CAD build for the part. Positions are in the model's coordinates, mm. Face numbers are marked on the shaded views. A direction names the side the tool comes from. Give positions to 0.01 mm unless a question says otherwise; leave off trailing zeros. Loops run counter-clockwise (first coordinate to the right, second up) from the corner with the lowest first, then second, coordinate; pieces in that order, holes last. Notation, with made-up numbers: (-27.5, 18.25) -> (7.5, 18.25) arc R35 ccw to (7.5, 52.25) -> close; hole circle Ø8 at (-24, -26). An arc over 180 degrees is marked (long way). Write each question's results on one line, items separated by ' | '. Start each with the question number.
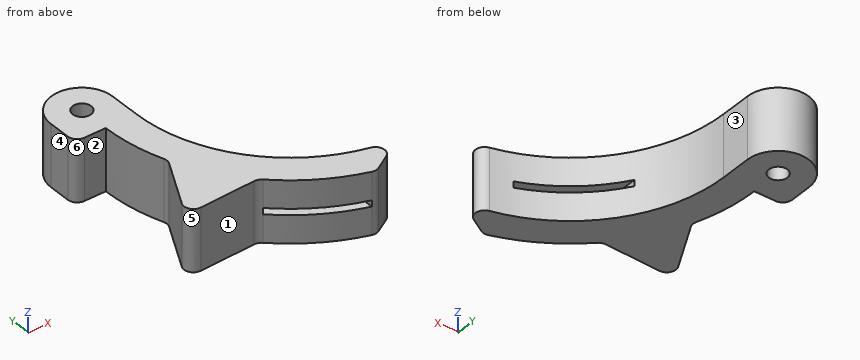
```python
from build123d import *

# Parameters (mm, degrees)
SKETCH_2_R              = 1.5
EXTRUDE_1_DEPTH         = 10
FILLET_1_R              = 1.5
CUT_EXTRUDE_START       = 8.978636738
CUT_EXTRUDE_6_OUTLINE_W = 18
CUT_EXTRUDE_6_OUTLINE_H = 1
CUT_EXTRUDE_6_DEPTH     = 12.065744551


# Read off the part's stored shape, not the designer's step: 切除-拉伸6
with BuildPart() as part:
    # 草图2 → 凸台-拉伸1 (new body)
    with BuildSketch(Plane.XY):
        with BuildLine():
            Line((-3.738313135, -26.487804482), (8.522639585, -25.945713856))
            ThreePointArc((8.522639585, -25.945713856), (14.597644225, -30.744268797), (21.698305683, -33.828489568))
            Line((21.698305683, -33.828489568), (28.148131868, -29.931317342))
            ThreePointArc((28.148131868, -29.931317342), (11.679291726, -22.010339454), (5, -5))
            Line((5, -5), (5, 0))
            ThreePointArc((5, 0), (0, 5), (-5, 0))
            Line((-5, 0), (-5, -5))
            Line((-5, -5), (1.011e-06, -5))
            ThreePointArc((1.011e-06, -5), (0.486326168, -10.379869542), (1.929534162, -15.585314685))
            Line((1.929534162, -15.585314685), (-3.738313135, -26.487804482))
        make_face()
        Circle(SKETCH_2_R, mode=Mode.SUBTRACT)
    extrude(amount=EXTRUDE_1_DEPTH)

    # 圆角1
    fillet_1_edges = [part.edges().sort_by_distance(p)[0] for p in [
        (-3.738313135, -26.487804482, 5),
        (1.929534162, -15.585314685, 5),
        (-5, -5, 5),
        (28.148131868, -29.931317342, 5),
        (21.698305683, -33.828489568, 5),
        (8.522639585, -25.945713856, 5),
    ]]
    fillet(fillet_1_edges, radius=FILLET_1_R)

    # 切除-拉伸6 outline → 切除-拉伸6 (cut)
    with BuildSketch(Plane.YZ.offset(CUT_EXTRUDE_START)):
        with Locations((-26, 5)):
            Rectangle(CUT_EXTRUDE_6_OUTLINE_W, CUT_EXTRUDE_6_OUTLINE_H)
    extrude(amount=CUT_EXTRUDE_6_DEPTH, mode=Mode.SUBTRACT)


solid = part.part
```
Q1. Drop flat-ended pins along their axis: pin 1 (0.8 mm diameter, centred on y = -30.5, z = 5, fed in from -X); pin 2 (1.5 mm diameter, centred on y = -25, z = 8, fed in from +X); pin 3 (1.5 mm diameter, centred on y = -2.5, z = 5.5, fed in from +X). Give the stop position or say it passes through.
Q2. Saw through at A-A, the plane z = 8.75. List the corners of the cut face in (x, y).
Q3. Saw through at C-C, the plane y = -1. List the corners of the cut face in (x, z).
Q4. Which spindle directions (+Z, -Z, +X, -X, +Y, -Y) get a long thin tool onto all of the face, cutting with end or side? Do the marked faces 1, 2 and 3. Say none if no direction does.
Q5. Saw through at D-D, the plane x = 12. List the corners of the cut face in (y, z).
Q6. Wall check: L1, parallel to Y at x = 2, z = 1.25; L2, parallel to X at y = -14.5, z = 1.75; L3, parallel to Y at x = 10.5, z = 1.5. Give the ranges that are in metal, low to high.
Q7. Saw through at B-B, the plane x = -0.5. List the corners of the cut face in (y, z), then the cut area to 3 significant figures.
Q8. Mould opens along Y. For the marked faces 4, 5 and 6 say: pulls with the +Y half, pulls with the -Y half, needs draft (parallel to the pull), parting line crosses it, or undercut.
Answer block:
1) pin 1: stops at x = 21.04 | pin 2: stops at x = 16.06 | pin 3: stops at x = 5
2) outline: (-5, -3.5) arc R1.5 ccw to (-3.5, -5) -> (0, -5) arc R30 ccw to (1.71, -14.98) arc R1.5 cw to (1.63, -16.17) -> (-2.54, -24.18) arc R1.5 ccw to (-1.14, -26.37) -> (7.86, -25.97) arc R1.5 cw to (8.98, -26.4) arc R30 ccw to (21.04, -33.63) arc R1.5 ccw to (22.27, -33.48) -> (24.62, -32.06) arc R1.5 ccw to (24.2, -29.32) arc R25 cw to (5, -5) -> (5, 0) arc R5 ccw to (-5, 0) -> close; hole circle Ø3 at (0, 0)
3) outline: (-5, 0) -> (-1.12, 0) -> (-1.12, 10) -> (-5, 10) -> close; (1.12, 0) -> (5, 0) -> (5, 10) -> (1.12, 10) -> close
4) face 1: +Z, -Z, -Y | face 2: +Z, -Z, -X | face 3: +Z, -Z, +X, +Y
5) outline: (-29, 0) -> (-22.35, 0) -> (-22.35, 4.5) -> (-29, 4.5) -> close; (-29, 5.5) -> (-22.35, 5.5) -> (-22.35, 10) -> (-29, 10) -> close
6) L1: y = -26.23 to 4.58 | L2: x = 1.54 to 6.88 | L3: y = -27.8 to -20.64
7) outline: (-26.34, 0) -> (-20.26, 0) -> (-20.26, 10) -> (-26.34, 10) -> close; (-5, 0) -> (-1.41, 0) -> (-1.41, 10) -> (-5, 10) -> close; (1.41, 0) -> (4.97, 0) -> (4.97, 10) -> (1.41, 10) -> close | area: 132 mm2
8) face 4: needs draft | face 5: undercut | face 6: pulls with the -Y half
